Design review of the part built by this model. Coordinates are the model's own, in mm. A direction names the side the tool comes from. Coordinates: 2 decimals unless noted, no trailing zeros. One line per item, written item: value. Start each with the question number.
1. Insertion check: pin 1 (10 mm diameter, centred on x = -28, z = 11.5, fed in from +Y); pin 2 (4 mm diameter, centred on y = 3, z = 14.5, fed in from +X); pin 3 (12 mm diameter, centred on x = 23.5, y = -12, fed in from -Z). Each pin has a flat end and moves straight along its axis. Give the tip position at first contact, or say it passes through.
2. Machinability: for faces 5 (the flat face through (0, 3, 19.5)), 6 (the cylindrical face through (-21.363, 10.782, 16.598)), 7 (the cylindrical face through (-0.534, 4.065, 33.955)), 8 (the flat face through (0, 48, 3.6)), which of the approach directions +Z, -Z, +X, -X, +Y, -Y give a long, thin tool a straight path to every point of the face, cutting with its end or side? Answer none if there is none.
3. Draft analysis for pull direction Z (two halves, no side actions). For faces 1 (the flat face through (-3, 0, 22.5)), 2 (the cylindrical face through (2.44, 0.54, 21.02)), 3 (the flat face through (-34, -33, 0.8)), 4 (the flat face through (17, 42, 6)), state which applies: pulls with the +Z half, pulls with the -Z half, needs draft (parallel to the pull), parting line crosses it, or undercut.
4. For probe 1 along X at (y, z) = (-2, 14) (3 decimals); probe 2 along Z at (x, y) = (-1, 7); probe 3 along X at (y, z) = (0, 2.5), list the stretches that pass through material, from the lowest coordinate up.
```python
from build123d import *

# Parameters (mm, degrees)
F2_R      = 20
F3_DEPTH  = 25
F4_R      = 2.5
F5_DEPTH  = 25
F7_W      = 12
F7_H      = 6.6
F8_DEPTH  = 60
F9_R      = 4.1
F9_R_2    = 2.5
F10_DEPTH = 15


# Not quite as in the source:
# - a fillet or chamfer that OpenCascade refuses, or shapes differently, is made with other operations: its cross-section is extruded or revolved along the edge and cut away or added
# - a feature names something its author has since deleted; it is built from what else it names


with BuildPart() as f1:
    # F0 (on Right) → F1 (revolve)
    with BuildSketch(Plane.YZ):
        with BuildLine():
            Line((-47, 0.8), (-47, 2))
            Line((-47, 2), (-47, 4))
            Line((-47, 4), (-42, 4))
            Line((-42, 4), (-42, 6))
            ThreePointArc((-42, 6), (-27.3273562245, 14.6498550341), (-11, 19.5))
            Line((-11, 19.5), (-2.5, 19.5))
            Line((-2.5, 19.5), (-2.5, 22.5))
            Line((-2.5, 22.5), (-11, 22.5))
            ThreePointArc((-11, 22.5), (-7.9199859369, 30.2852233625), (0, 33))
            Line((0, 33), (0, 36))
            ThreePointArc((0, 36), (-9.9253616904, 31.873751261), (-14, 21.9270907164))
            ThreePointArc((-14, 21.9270907164), (-30.5537547763, 16.0145412775), (-45, 6))
            Line((-45, 6), (-50, 6))
            Line((-50, 6), (-50, 0.8))
            Line((-50, 0.8), (-47, 0.8))
        make_face()
    revolve(axis=Axis((0, 0, -9), (0, 0, -1)))

    # F2 (on Top) → F3 (cut)
    with BuildSketch(Plane.XY):
        Circle(F2_R)
    extrude(amount=-F3_DEPTH, mode=Mode.SUBTRACT)

    # F4 (on Top) → F5 (cut)
    with BuildSketch(Plane.XY):
        with Locations((0, -26)):
            Circle(F4_R)
        with Locations((-22.5166604984, 13)):
            Circle(F4_R)
        with Locations((22.5166604984, 13)):
            Circle(F4_R)
    extrude(amount=F5_DEPTH, mode=Mode.SUBTRACT)

    # F6: fillet of radius 5 on 1 edges, made by hand

    # F6_s1 → F6_t2 (revolve)
    with BuildSketch(Plane.YZ):
        with BuildLine():
            ThreePointArc((-42, 4), (-41.3412296148, 5.9882107587), (-39.9258684636, 7.532138624))
            ThreePointArc((-39.9258684636, 7.532138624), (-40.9699899366, 6.7756209672), (-42, 6))
            Line((-42, 6), (-42, 4))
        make_face()
    revolve(axis=Axis((0, 0, 6), (0, 0, -1)))

    # F7 (on Front) → F8 (cut)
    with BuildSketch(Plane.XZ):
        with Locations((0, 0.3)):
            Rectangle(F7_W, F7_H)
    extrude(amount=-F8_DEPTH, mode=Mode.SUBTRACT)

    # F9 (on face) → F10 (cut)
    with BuildSketch(Plane.XY.offset(22.5)):
        Circle(F9_R)
        Circle(F9_R_2, mode=Mode.SUBTRACT)
        Circle(F9_R_2)
    extrude(amount=F10_DEPTH, mode=Mode.SUBTRACT)

    # F11: fillet of radius 2.5 on 2 edges, made by hand

    # F11_s1 → F11_t2 (revolve)
    with BuildSketch(Plane.YZ):
        with BuildLine():
            ThreePointArc((-15.7934154108, 21.5162006837), (-14.513888258, 22.2873217713), (-13.902565029, 23.6504436939))
            ThreePointArc((-13.902565029, 23.6504436939), (-13.9778675149, 22.7902702686), (-14, 21.9270907164))
            ThreePointArc((-14, 21.9270907164), (-14.8981182002, 21.7278020994), (-15.7934154108, 21.5162006837))
        make_face()
    revolve(axis=Axis((0, 0, 21.9270907164), (0, 0, -1)))

    # F11_s3 → F11_t4 (revolve, cut)
    with BuildSketch(Plane.YZ):
        with BuildLine():
            ThreePointArc((-47.5, 6), (-49.267766953, 5.267766953), (-50, 3.5))
            Line((-50, 3.5), (-50, 6))
            Line((-50, 6), (-47.5, 6))
        make_face()
    revolve(axis=Axis((0, 0, 6), (0, 0, -1)), mode=Mode.SUBTRACT)


solid = f1.part
```
Worked answers:
1. pin 1: stops at y = 35.47
1. pin 2: stops at x = 36.48
1. pin 3: stops at z = 12.2
2. face 5: -Z
2. face 6: +Z, -Z
2. face 7: +Z
2. face 8: -Z, +Y
3. face 1: undercut
3. face 2: needs draft
3. face 3: pulls with the -Z half
3. face 4: pulls with the +Z half
4. probe 1: x = -34.134 to -28.705, 28.705 to 34.134
4. probe 2: z = 19.5 to 22.5, 31.01 to 34.08
4. probe 3: x = -50 to -47, 47 to 50
